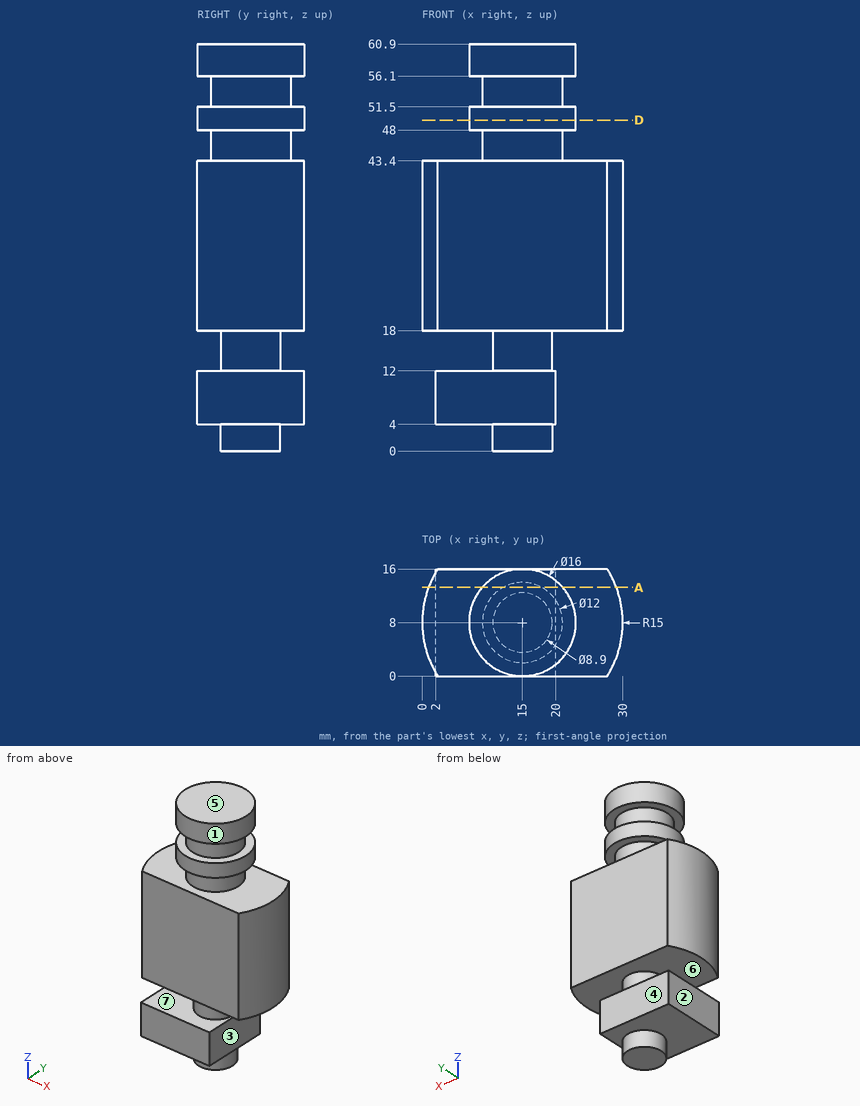
Could you check a few things on this drawing? It's one solid part, dimensions in mm from its lowest x, y, z. A direction names the side the tool comes from. Coordinates: 2 decimals unless noted, no trailing zeros. Loops run counter-clockwise (first coordinate to the right, second up) from the corner with the lowest first, then second, coordinate; pieces in that order, holes last.
1. Imagine slicing it at D-D (z = 49.5). Please give me the cut outline in (x, y), and give its area (3 significant figures).
2. I need wall thicknesses on L1, parallel to Z at x = 13, y = 2; L2, parallel to Z at x = 11, y = 11; L3, parallel to Z at x = 2.5, y = 3.5. Which ranges of each line are inside material? Lowest first, please.
3. Imagine slicing it at A-A (y = 13.25). Please give me the cut outline in (x, z), and give its area (3 significant figures).
4. We'd pull the mould along Z, two halves only. Please class the marked faces 4, 5, 6 and 7: released by +Z, released by -Z, zero draft, split by the parting line, or undercut.
5. For the marked faces 1, 2 and 3, which set-ups out of +Z, -Z, +X, -X, +Y, -Y let a thin tool reach every point of the face, with its end or its side?
6. For P1, Ø8, axis at x = 19, y = 8.5, coming from the -Z side; P2, Ø6, axis at x = 20.5, y = 2.5, coming from the -Z side; P3, Ø1.5, axis at y = 10.5, z = 20.5, coming from the -X side; P4, Ø1.5, axis at y = 2, z = 13.5, coming from the +X side, each with a flat end and sliding along its axis, tell me the tip position at first contact or that it passes through.
Computed values:
1. outline: circle Ø16 at (15, 8)
1. area: 201 mm2
2. L1: z = 4 to 12, 18 to 43.4, 48 to 51.5, 56.1 to 60.9
2. L2: z = 4 to 12, 18 to 60.9
2. L3: z = 4 to 12, 18 to 43.4
3. outline: (0.95, 18) - (29.05, 18) - (29.05, 43.4) - (17.9, 43.4) - (17.9, 48) - (21.04, 48) - (21.04, 51.5) - (17.9, 51.5) - (17.9, 56.1) - (21.04, 56.1) - (21.04, 60.9) - (8.96, 60.9) - (8.96, 56.1) - (12.1, 56.1) - (12.1, 51.5) - (8.96, 51.5) - (8.96, 48) - (12.1, 48) - (12.1, 43.4) - (0.95, 43.4) - close; (2, 4) - (20, 4) - (20, 12) - (2, 12) - close
3. area: 1,010 mm2
4. face 4: zero draft
4. face 5: released by +Z
4. face 6: undercut
4. face 7: undercut
5. face 1: +Z
5. face 2: -Z, -X, +Y, -Y
5. face 3: -Z, +X, +Y, -Y
6. P1: stops at z = 0
6. P2: stops at z = 4
6. P3: stops at x = 0.1
6. P4: passes through
